Read the model definition and answer for the solid it produces. Units are mm, in the model's axes. A direction names the side the tool comes from. Coordinates: 2 decimals unless noted, no trailing zeros. Write each loop counter-clockwise with the first axis right and the second up, starting at its lowest first coordinate (ties: lowest second). Pieces come first, ordered by that corner, then holes. Notation, with made-up numbers: (-3.5, -36.5) - (7.5, -36.5) arc R13 cw to (7.5, -19.5) - close; hole circle Ø8 at (-1, -32). An arc over 180 degrees is marked (long way). Return JSON: item names as keys, results as strings.
```python
from build123d import *

# Parameters (mm, degrees)
SKETCH1_W           = 10
SKETCH1_H           = 3
BOSS_EXTRUDE1_DEPTH = 3
FILLET1_R           = 0.25


with BuildPart() as part:
    # Sketch1 → Boss-Extrude1 (new body)
    with BuildSketch(Plane.XY):
        with BuildLine():
            Line((34.843392212, -14.218278754), (31.843392212, -14.218278754))
            Line((31.843392212, -14.218278754), (31.843392212, -13.218278754))
            ThreePointArc((31.843392212, -13.218278754), (32.043392212, -12.218278754), (31.843392212, -11.218278754))
            Line((31.843392212, -11.218278754), (31.843392212, 11.781721246))
            Line((31.843392212, 11.781721246), (37.843392212, 11.781721246))
            Line((37.843392212, 11.781721246), (37.843392212, 21.781721246))
            Line((37.843392212, 21.781721246), (34.843392212, 21.781721246))
            Line((34.843392212, 21.781721246), (34.843392212, 20.781721246))
            ThreePointArc((34.843392212, 20.781721246), (34.643392212, 19.781721246), (34.843392212, 18.781721246))
            Line((34.843392212, 18.781721246), (34.843392212, 17.781721246))
            Line((34.843392212, 17.781721246), (31.843392212, 17.781721246))
            Line((31.843392212, 17.781721246), (31.843392212, 18.781721246))
            ThreePointArc((31.843392212, 18.781721246), (32.043392212, 19.781721246), (31.843392212, 20.781721246))
            Line((31.843392212, 20.781721246), (31.843392212, 21.781721246))
            Line((31.843392212, 21.781721246), (-34.256607788, 21.781721246))
            Line((-34.256607788, 21.781721246), (-34.256607788, 20.781721246))
            ThreePointArc((-34.256607788, 20.781721246), (-34.456607788, 19.781721246), (-34.256607788, 18.781721246))
            Line((-34.256607788, 18.781721246), (-34.256607788, 17.781721246))
            Line((-34.256607788, 17.781721246), (-37.256607788, 17.781721246))
            Line((-37.256607788, 17.781721246), (-37.256607788, 18.781721246))
            ThreePointArc((-37.256607788, 18.781721246), (-37.056607788, 19.781721246), (-37.256607788, 20.781721246))
            Line((-37.256607788, 20.781721246), (-37.256607788, 21.781721246))
            Line((-37.256607788, 21.781721246), (-40.256607788, 21.781721246))
            Line((-40.256607788, 21.781721246), (-40.256607788, 11.781721246))
            Line((-40.256607788, 11.781721246), (-34.256607788, 11.781721246))
            Line((-34.256607788, 11.781721246), (-34.256607788, -11.218278754))
            ThreePointArc((-34.256607788, -11.218278754), (-34.456607788, -12.218278754), (-34.256607788, -13.218278754))
            Line((-34.256607788, -13.218278754), (-34.256607788, -14.218278754))
            Line((-34.256607788, -14.218278754), (-37.256607788, -14.218278754))
            Line((-37.256607788, -14.218278754), (-37.256607788, -13.218278754))
            ThreePointArc((-37.256607788, -13.218278754), (-37.056607788, -12.218278754), (-37.256607788, -11.218278754))
            Line((-37.256607788, -11.218278754), (-37.256607788, -10.218278754))
            Line((-37.256607788, -10.218278754), (-40.256607788, -10.218278754))
            Line((-40.256607788, -10.218278754), (-40.256607788, -26.218278754))
            Line((-40.256607788, -26.218278754), (37.843392212, -26.218278754))
            Line((37.843392212, -26.218278754), (37.843392212, -10.218278754))
            Line((37.843392212, -10.218278754), (34.843392212, -10.218278754))
            Line((34.843392212, -10.218278754), (34.843392212, -11.218278754))
            ThreePointArc((34.843392212, -11.218278754), (34.643392212, -12.218278754), (34.843392212, -13.218278754))
            Line((34.843392212, -13.218278754), (34.843392212, -14.218278754))
        make_face()
        with Locations((-1.206607788, -21.718278754)):
            Rectangle(SKETCH1_W, SKETCH1_H, mode=Mode.SUBTRACT)
        with Locations((18.793392212, -21.718278754)):
            Rectangle(SKETCH1_W, SKETCH1_H, mode=Mode.SUBTRACT)
        with Locations((-21.206607788, -21.718278754)):
            Rectangle(SKETCH1_W, SKETCH1_H, mode=Mode.SUBTRACT)
    extrude(amount=BOSS_EXTRUDE1_DEPTH)

    # Fillet1
    fillet1_edges = [part.edges().sort_by_distance(p)[0] for p in [
        (34.843392212, 21.781721246, 1.5),
        (34.843392212, -10.218278754, 1.5),
        (-37.256607788, -10.218278754, 1.5),
        (-37.256607788, 21.781721246, 1.5),
    ]]
    fillet(fillet1_edges, radius=FILLET1_R)


solid = part.part
```
(1) A cutting plane is placed at C-C (z = 1.3). State how many separate pieces and enclosed holes the cut face has, and give its area (3 significant figures).
Answer:
{"separate pieces": "1", "enclosed holes": "3", "area": "3,350 mm²"}
(2) Determine the mould class of faces 1 (the face through (-37.057, -12.233, 1.479)), 2 (the face through (-2, -26.218, 1)) for opening direction X: +X half, -X half, draft (parallel to the pull), parting line (faces both ways), or undercut.
Answer:
{"face 1": "undercut", "face 2": "draft"}
(3) A cutting plane is placed at A-A (x = 1). Determine the outline of the cut face in (y, z), and give its area (3 significant figures).
Answer:
{"outline": "(-26.22, 0) - (-23.22, 0) - (-23.22, 3) - (-26.22, 3) - close; (-20.22, 0) - (21.78, 0) - (21.78, 3) - (-20.22, 3) - close", "area": "135 mm²"}
(4) Straight lines are drawn through the part: line 1 (X direction, y = -21.5, z = 1.7); line 2 (Y direction, x = 18.5, z = 2); line 3 (X direction, y = -11, z = 1.45). For each, find the intervals that lie inside material, in ascending order. Write a range as from..to.
Answer:
{"line 1": "-40.26..-26.21, -16.21..-6.21, 3.79..13.79, 23.79..37.84", "line 2": "-26.22..-23.22, -20.22..21.78", "line 3": "-40.26..-37.26, -34.26..31.84, 34.84..37.84"}
(5) A cutting plane is placed at D-D (y = 7). Determine the outline of the cut face in (x, z).
Answer:
{"outline": "(-34.26, 0) - (31.84, 0) - (31.84, 3) - (-34.26, 3) - close"}
(6) Which of the six approach directions +Z, -Z, +X, -X, +Y, -Y give full straight-line access (tool end or side, diameter ignored) to faces 3 (the face through (36, -10.218, 1)), 4 (the face through (-2, -2, 0)), 5 (the face through (-36, -14.218, 1))?
Answer:
{"face 3": "+Z, -Z, +X", "face 4": "-Z, +X, -X, +Y, -Y", "face 5": "+Z, -Z"}
(7) A cutting plane is placed at B-B (x = 33). Determine the outline of the cut face in (y, z), and give its area (3 significant figures).
Answer:
{"outline": "(-26.22, 0) - (-14.22, 0) - (-14.22, 3) - (-26.22, 3) - close; (11.78, 0) - (17.78, 0) - (17.78, 3) - (11.78, 3) - close", "area": "54.0 mm²"}
